Source: CAD feature listing. Evaluate the final solid. Frame: model axes, mm. Face numbers are marked on the shaded views. A direction names the side the tool comes from. Round coordinates to 2 decimals unless told otherwise and drop trailing zeros. Loops run counter-clockwise (first coordinate to the right, second up) from the corner with the lowest first, then second, coordinate; pieces in that order, holes last. Notation, with made-up numbers: (75, -14) -> (115, -14) arc R15 ccw to (115, -6) -> close; hole circle Ø6 at (86.25, -24). An arc over 180 degrees is marked (long way). Put each result on its own line as item: value. Start each with the question number.
1. Contact query for flat-ended pins moving along their axis: pin 1 (0.5 mm diameter, centred on x = 11, z = 0.5, fed in from +Y); pin 2 (1.8 mm diameter, centred on x = 22, y = 23, fed in from -Z); pin 3 (2 mm diameter, centred on x = 22.5, z = -0.5, fed in from +Y). Output: stop coordinate, or through.
2. Cut plane B-B (y = 10). Return the cut outline in (x, z), then the cut area to 3 significant figures.
3. Set-up query: the marked faces 1, 2 and 3. Return all of +Z, -Z, +X, -X, +Y, -Y with unobstructed straight access to the full face (end or side cutting, diameter ignored); none if empty.
4. Cut plane D-D (z = -3.4). Return the cut outline in (x, y), then the cut area to 3 significant figures.
5. Draft query along X for the marked faces 4, 5, 6 and 7. Return one class per face: pulls with the +X half, pulls with the -X half, needs draft (parallel to the pull), parting line crosses it, or undercut.
6. Cut plane C-C (x = 34). Return the cut outline in (y, z), then the cut area to 3 significant figures.
7. Cut plane A-A (z = 0.55). Return the cut outline in (x, y).
8. Material intervals for L1, parallel to Y at x = 4, z = -2.9; L2, parallel to X at y = 4.25, z = -0.1; L3, parallel to X at y = 12.25, z = -3, sorted ascending.
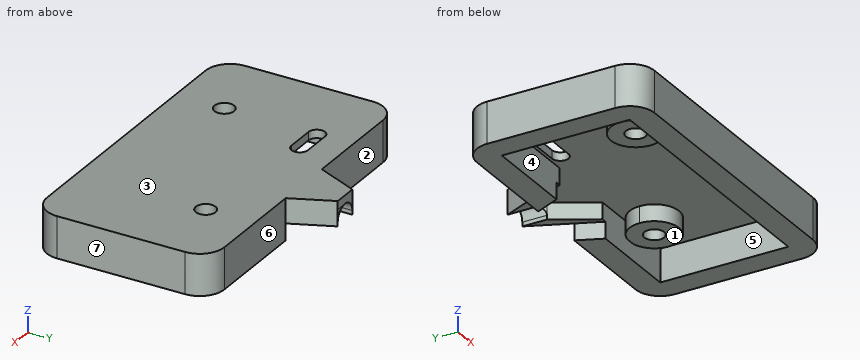
```python
from build123d import *

# Parameters (mm, degrees)
SKICA1_W                 = 38.5
SKICA1_H                 = 21.5
P_IDAT_VYSUNUT_M1_DEPTH  = 1
SKICA2_W                 = 38.5
SKICA2_H                 = 21.5
SKICA2_W_2               = 32.5
SKICA2_H_2               = 15.5
P_IDAT_VYSUNUT_M2_DEPTH  = 4
ZAOBLIT1_R               = 3
SKICA3_R                 = 1.2
ODEBRAT_VYSUNUT_M1_DEPTH = 2
SKICA4_R                 = 1.2
P_IDAT_VYSUNUT_M5_DEPTH  = 2
ODEBRAT_VYSUNUT_M2_DEPTH = 2
P_IDAT_VYSUNUT_M6_DEPTH  = 1
P_IDAT_VYSUNUT_M7_DEPTH  = 2
ODEBRAT_VYSUNUT_M5_DEPTH = 2
SKICA10_W                = 3
SKICA10_H                = 3
ODEBRAT_VYSUNUT_M6_DEPTH = 2
ZKOSEN_2_SIZE            = 2.886751346
ZKOSEN_2_SIZE_2          = 5
ZKOSEN_3_SIZE            = 2.886751346
ZKOSEN_3_SIZE_2          = 5
ZAOBLIT4_R               = 1.5


with BuildPart() as part:
    # Skica1 → Přidat vysunutím1 (new body)
    with BuildSketch(Plane.XY):
        with Locations((19.25, 10.75)):
            Rectangle(SKICA1_W, SKICA1_H)
    extrude(amount=P_IDAT_VYSUNUT_M1_DEPTH)

    # Skica2 → Přidat vysunutím2 (add)
    with BuildSketch(Plane(origin=(0, 0, 0), x_dir=(-1, 0, 0), z_dir=(0, 0, -1))):
        with Locations((-19.25, 10.75)):
            Rectangle(SKICA2_W, SKICA2_H)
        with Locations((-19.25, 10.75)):
            Rectangle(SKICA2_W_2, SKICA2_H_2, mode=Mode.SUBTRACT)
    extrude(amount=P_IDAT_VYSUNUT_M2_DEPTH)

    # Zaoblit1
    zaoblit1_edges = [part.edges().sort_by_distance(p)[0] for p in [
        (0, 0, -1.5),
        (38.5, 0, -1.5),
        (38.5, 21.5, -1.5),
        (0, 21.5, -1.5),
    ]]
    fillet(zaoblit1_edges, radius=ZAOBLIT1_R)

    # Skica3 → Odebrat vysunutím1 (cut)
    with BuildSketch(Plane.XY.offset(1)):
        with Locations((9.166704, 5.920968857)):
            Circle(SKICA3_R)
        with Locations((29.333296, 15.579031143)):
            Circle(SKICA3_R)
    extrude(amount=-ODEBRAT_VYSUNUT_M1_DEPTH, mode=Mode.SUBTRACT)

    # Skica4 → Přidat vysunutím5 (add)
    # profile 1 of 2: a face of its own
    with BuildSketch(Plane(origin=(0, 0, 0), x_dir=(-1, 0, 0), z_dir=(0, 0, -1))):
        with BuildLine():
            ThreePointArc((-30.017358084, 18.5), (-31.197137966, 13.228266772), (-26.333296, 15.579031143))
            ThreePointArc((-26.333296, 15.579031143), (-26.98253163, 17.442873109), (-28.649233916, 18.5))
            Line((-28.649233916, 18.5), (-30.017358084, 18.5))
        make_face()
        with Locations(Location((-29.333296, 15.579031143, 0), (0, 0, 180))):
            Circle(SKICA4_R, mode=Mode.SUBTRACT)
    # profile 2 of 2: a face of its own
    with BuildSketch(Plane(origin=(0, 0, 0), x_dir=(-1, 0, 0), z_dir=(0, 0, -1))):
        with BuildLine():
            ThreePointArc((-8.482641916, 3), (-6.81593963, 4.057126891), (-6.166704, 5.920968857))
            ThreePointArc((-6.166704, 5.920968857), (-11.030545966, 8.271733228), (-9.850766084, 3))
            Line((-9.850766084, 3), (-8.482641916, 3))
        make_face()
        with Locations(Location((-9.166704, 5.920968857, 0), (0, 0, 180))):
            Circle(SKICA4_R, mode=Mode.SUBTRACT)
    extrude(amount=P_IDAT_VYSUNUT_M5_DEPTH)

    # Skica5 → Odebrat vysunutím2 (cut)
    with BuildSketch(Plane.XY.offset(1)):
        with BuildLine():
            Line((9.166704, 18.120968857), (12.666704, 18.120968857))
            ThreePointArc((12.666704, 18.120968857), (13.666704, 17.120968857), (12.666704, 16.120968857))
            Line((12.666704, 16.120968857), (9.166704, 16.120968857))
            ThreePointArc((9.166704, 16.120968857), (8.166704, 17.120968857), (9.166704, 18.120968857))
        make_face()
    extrude(amount=-ODEBRAT_VYSUNUT_M2_DEPTH, mode=Mode.SUBTRACT)

    # Skica7 → Přidat vysunutím6 (add)
    with BuildSketch(Plane.XY.offset(1)):
        Polygon((15.55, 21.5), (17.75, 26.5), (20.75, 26.5), (22.95, 21.5), align=None)
    extrude(amount=-P_IDAT_VYSUNUT_M6_DEPTH)

    # Skica8 → Přidat vysunutím7 (add)
    with BuildSketch(Plane(origin=(0, 0, 0), x_dir=(-1, 0, 0), z_dir=(0, 0, -1))):
        Polygon((-15.55, 21.5), (-17.75, 26.5), (-17.75, 21.5), align=None)
        Polygon((-20.75, 26.5), (-22.95, 21.5), (-20.75, 21.5), align=None)
    extrude(amount=P_IDAT_VYSUNUT_M7_DEPTH)

    # Skica9 → Odebrat vysunutím5 (cut)
    with BuildSketch(Plane(origin=(0, 0, -4), x_dir=(-1, 0, 0), z_dir=(0, 0, -1))):
        Polygon((-22.95, 21.5), (-24.27, 18.5), (-14.23, 18.5), (-15.55, 21.5), align=None)
    extrude(amount=-ODEBRAT_VYSUNUT_M5_DEPTH, mode=Mode.SUBTRACT)

    # Skica10 → Odebrat vysunutím6 (cut)
    with BuildSketch(Plane(origin=(0, 0, -2), x_dir=(-1, 0, 0), z_dir=(0, 0, -1))):
        with Locations((-19.25, 20)):
            Rectangle(SKICA10_W, SKICA10_H)
    extrude(amount=-ODEBRAT_VYSUNUT_M6_DEPTH, mode=Mode.SUBTRACT)

    # Zkosení2
    # the kernel refuses this chamfer: 5, 2.886751346 mm, written as the material it takes off along each edge
    with BuildSketch(Plane(origin=(20.75, 18.5, -14.935428773), x_dir=(0.9983227437537926, -0.057893862402670485, 0), z_dir=(0, 0, 1))) as zkosen_2_piece_1:
        Polygon((ZKOSEN_2_SIZE * 0.998322743736, ZKOSEN_2_SIZE * 0.0578938624016), (-ZKOSEN_2_SIZE_2 * 0.0578938624027, ZKOSEN_2_SIZE_2 * 0.998322743754), (0, 0), align=None)
    extrude(amount=14.935428773, mode=Mode.SUBTRACT)

    # Zkosení3
    # the kernel refuses this chamfer: 5, 2.886751346 mm, written as the material it takes off along each edge
    with BuildSketch(Plane(origin=(17.75, 18.5, -14.935428773), x_dir=(-0.9983227437537926, -0.05789386240267058, 0), z_dir=(0, 0, 1))) as zkosen_3_piece_1:
        Polygon((ZKOSEN_3_SIZE * 0.998322743736, -ZKOSEN_3_SIZE * 0.0578938624016), (-ZKOSEN_3_SIZE_2 * 0.0578938624027, -ZKOSEN_3_SIZE_2 * 0.998322743754), (0, 0), align=None)
    extrude(amount=14.935428773, mode=Mode.SUBTRACT)

    # Zaoblit4
    # the kernel refuses this fillet: 1.5 mm, written as the material it adds along each edge
    with BuildSketch(Plane(origin=(17.75, 26.5, 0), x_dir=(1, 0, 0), z_dir=(0, -1, 0))) as zaoblit4_piece_1_section:
        with BuildLine():
            CenterArc((ZAOBLIT4_R, -ZAOBLIT4_R), ZAOBLIT4_R, 90, 90)
            Line((0, -ZAOBLIT4_R), (0, 0))
            Line((0, 0), (ZAOBLIT4_R, 0))
        make_face()
    zaoblit4_piece_1 = extrude(amount=6.75, mode=Mode.PRIVATE)
    zaoblit4_piece_1 = split(zaoblit4_piece_1, bisect_by=Plane(origin=(17.323921005, 25.531638648, -0.383561124), z_dir=(0.9153150324227655, -0.4027386142660173, 0)), keep=Keep.TOP, mode=Mode.PRIVATE)
    zaoblit4_piece_1 = split(zaoblit4_piece_1, bisect_by=Plane(origin=(18.56429614, 24.910402286, -0.383561124), z_dir=(-0.8660254037846095, 0.4999999999997042, 0)), keep=Keep.TOP, mode=Mode.PRIVATE)
    add(zaoblit4_piece_1)
    with BuildSketch(Plane(origin=(20.75, 19.75, 0), x_dir=(0, 0, -1), z_dir=(0, 1, 0))) as zaoblit4_piece_2_section:
        with BuildLine():
            CenterArc((ZAOBLIT4_R, ZAOBLIT4_R), ZAOBLIT4_R, 180, 90)
            Line((0, ZAOBLIT4_R), (0, 0))
            Line((0, 0), (ZAOBLIT4_R, 0))
        make_face()
    zaoblit4_piece_2 = extrude(amount=6.75, mode=Mode.PRIVATE)
    zaoblit4_piece_2 = split(zaoblit4_piece_2, bisect_by=Plane(origin=(21.176078995, 25.531638648, -0.383561124), z_dir=(-0.9153150324227657, -0.4027386142660168, 0)), keep=Keep.TOP, mode=Mode.PRIVATE)
    zaoblit4_piece_2 = split(zaoblit4_piece_2, bisect_by=Plane(origin=(19.93570386, 24.910402286, -0.383561124), z_dir=(0.8660254037846095, 0.4999999999997042, 0)), keep=Keep.TOP, mode=Mode.PRIVATE)
    add(zaoblit4_piece_2)


solid = part.part
```
Solution:
1. pin 1: stops at y = 21.5
1. pin 2: stops at z = -2
1. pin 3: stops at y = 24.8
2. outline: (0, -4) -> (3, -4) -> (3, 0) -> (35.5, 0) -> (35.5, -4) -> (38.5, -4) -> (38.5, 1) -> (0, 1) -> close
2. area: 62.5 mm^2
3. face 1: -Z
3. face 2: +Z, -Z, -X, +Y
3. face 3: +Z, +X, -X, +Y, -Y
4. outline: (0, 3) arc R3 ccw to (3, 0) -> (35.5, 0) arc R3 ccw to (38.5, 3) -> (38.5, 18.5) arc R3 ccw to (35.5, 21.5) -> (22.95, 21.5) -> (24.27, 18.5) -> (35.5, 18.5) -> (35.5, 3) -> (3, 3) -> (3, 18.5) -> (14.23, 18.5) -> (15.55, 21.5) -> (3, 21.5) arc R3 ccw to (0, 18.5) -> close
4. area: 290 mm^2
5. face 4: undercut
5. face 5: undercut
5. face 6: needs draft
5. face 7: pulls with the +X half
6. outline: (0, -4) -> (3, -4) -> (3, 0) -> (18.5, 0) -> (18.5, -4) -> (21.5, -4) -> (21.5, 1) -> (0, 1) -> close
6. area: 45.5 mm^2
7. outline: (0, 3) arc R3 ccw to (3, 0) -> (35.5, 0) arc R3 ccw to (38.5, 3) -> (38.5, 18.5) arc R3 ccw to (35.5, 21.5) -> (22.95, 21.5) -> (20.75, 26.5) -> (17.75, 26.5) -> (15.55, 21.5) -> (3, 21.5) arc R3 ccw to (0, 18.5) -> close; hole circle Ø2.4 at (9.17, 5.92); hole (9.17, 16.12) -> (12.67, 16.12) arc R1 ccw to (12.67, 18.12) -> (9.17, 18.12) arc R1 ccw to start; hole circle Ø2.4 at (29.33, 15.58)
8. L1: y = 0 to 3, 18.5 to 21.5
8. L2: x = 0 to 3, 6.68 to 11.66, 35.5 to 38.5
8. L3: x = 0 to 3, 35.5 to 38.5
